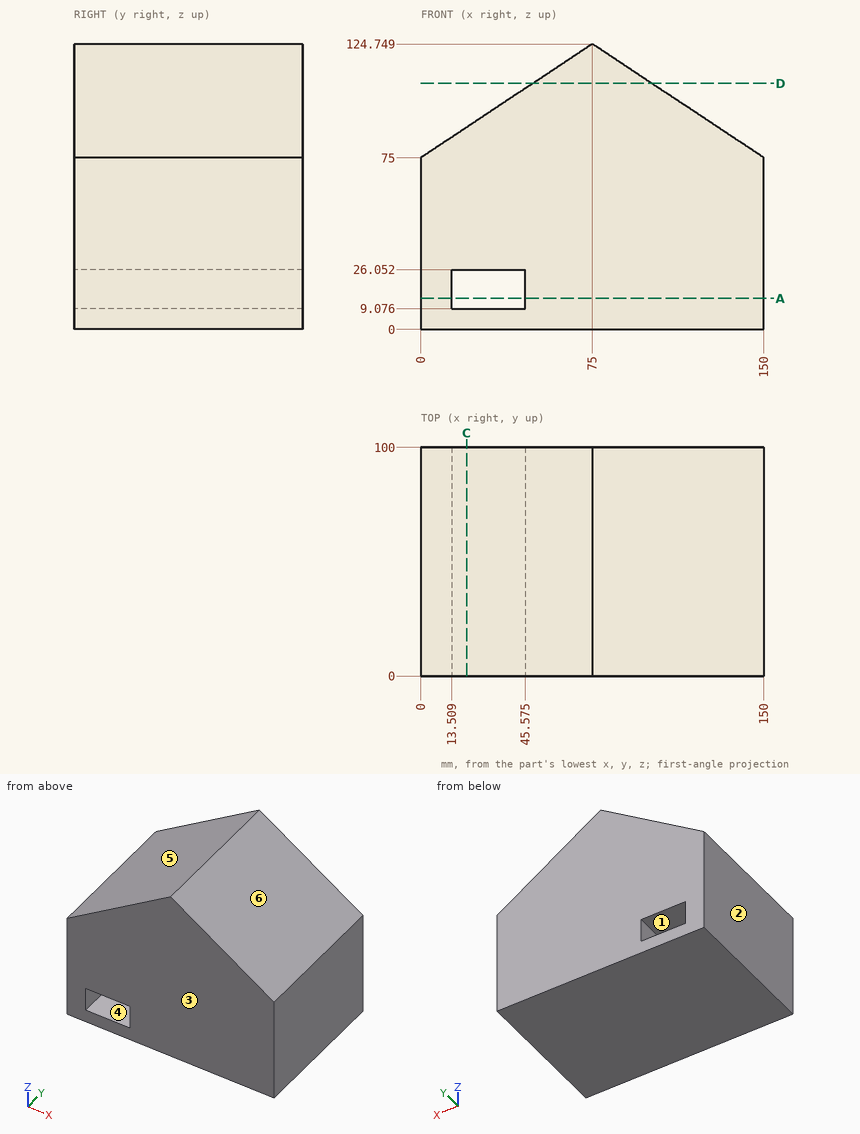
Geometry: see drawing. Coordinates: mm, zero at the bounding-box minimum. A direction names the side the tool comes from. Round coordinates to 2 decimals unless told otherwise and drop trailing zeros. Loops run counter-clockwise (first coordinate to the right, second up) from the corner with the lowest first, then second, coordinate; pieces in that order, holes last. Notation, with made-up numbers: M 28,22.5 L 51,22.5 A8 cw 51,29.5 Z; hole C 66.25,41.5 d6. An arc over 180 degrees is marked long. Use a Markdown table: item, result. Add a question column.
1. Section query C-C on x = 20. Return the cut outline in (y, z).
2. Contact query for flat-ended pins moving along their axis: P1, Ø3, axis at x = 21.5, y = 41, coming from the +Z side; P2, Ø5, axis at x = 105, z = 109, coming from the -Y side. Output: stop coordinate, or through.
3. Section query D-D on z = 107.5. Return the cut outline in (x, y) (1 decimal).
4. Line query: line 1 (X direction, y = 76.5, z = 17.5) (1 decimal); line 2 (Z direction, x = 32, y = 55) (1 decimal); line 3 (Z direction, x = 23, y = 60) (1 decimal). Output: solid intervals per line, ascending.
5. Section query A-A on z = 13.5. Return the cut outline in (x, y) (1 decimal), then the cut area to 3 significant figures.
6. Reachability of the marked faces 1 and 2 from +Z, -Z, +X, -X, +Y, -Y: full face, straight path, thin tool, end or side. Return the list, or none.
7. Mould query, pull axis X, two halves, no side actions, for the marked faces 3, 4, 5 and 6. Classes: pulls with the +X half, pulls with the -X half, needs draft (parallel to the pull), parting line crosses it, or undercut.
Reported:
| question | item | result |
|---|---|---|
| 1 | outline | M 0,0 L 100,0 L 100,9.08 L 0,9.08 Z; M 0,26.05 L 100,26.05 L 100,88.27 L 0,88.27 Z |
| 2 | P1 | stops at z = 90.26 |
| 2 | P2 | passes through |
| 3 | outline | M 49,0 L 101,0 L 101,100 L 49,100 Z |
| 4 | line 1 | x = 0 to 13.5, 45.6 to 150 |
| 4 | line 2 | z = 0 to 9.1, 26.1 to 96.2 |
| 4 | line 3 | z = 0 to 9.1, 26.1 to 90.3 |
| 5 | outline | M 0,0 L 13.5,0 L 13.5,100 L 0,100 Z; M 45.6,0 L 150,0 L 150,100 L 45.6,100 Z |
| 5 | area | 11,800 mm² |
| 6 | face 1 | +Y, -Y |
| 6 | face 2 | +Z, -Z, -X, +Y, -Y |
| 7 | face 3 | needs draft |
| 7 | face 4 | undercut |
| 7 | face 5 | pulls with the -X half |
| 7 | face 6 | pulls with the +X half |
